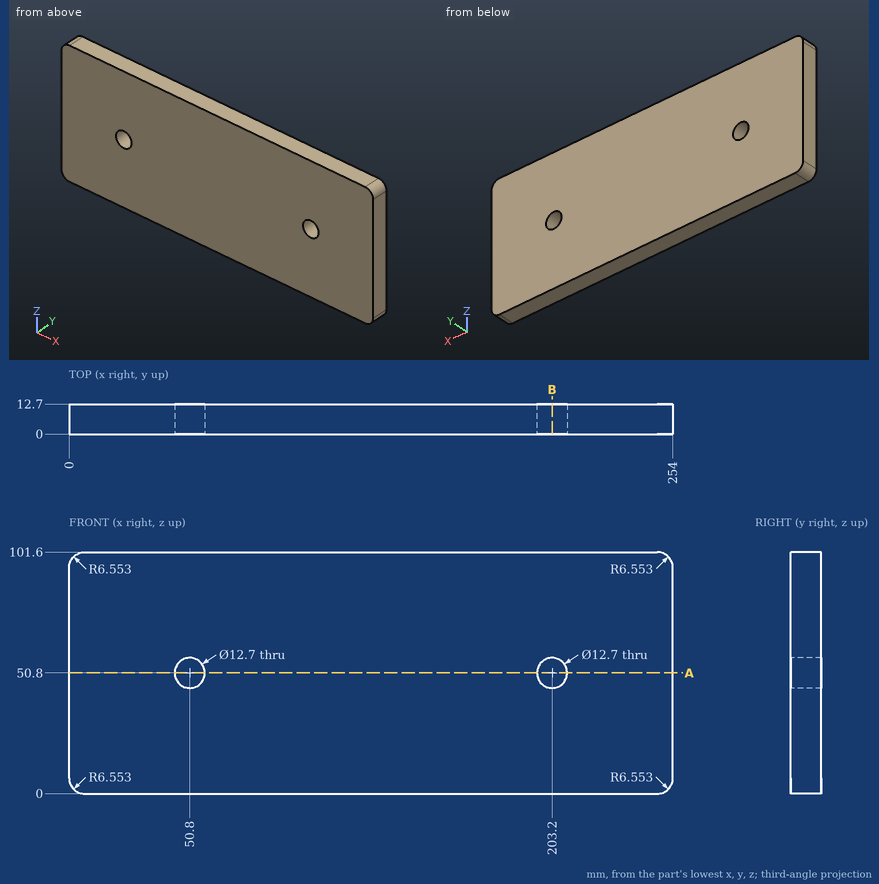
Source: three-view drawing plus pictorial views. Frame: mm from the lowest corner of the part. Round coordinates to 2 decimals unless told otherwise and drop trailing zeros. Loops run counter-clockwise (first coordinate to the right, second up) from the corner with the lowest first, then second, coordinate; pieces in that order, holes last. Notation, with made-up numbers: (2.25, -37) -> (49.25, -37) arc R18 cw to (49.25, -20) -> close; hole circle Ø11 at (-7, 55.25). An arc over 180 degrees is marked (long way). Use one line per item in the form item = value.
Item 1: Cut plane A-A on z = 50.8. Output: boundary loops of the cut face in (x, y).
Evaluation:
outline = (0, 0) -> (44.45, 0) -> (44.45, 12.7) -> (0, 12.7) -> close; (57.15, 0) -> (196.85, 0) -> (196.85, 12.7) -> (57.15, 12.7) -> close; (209.55, 0) -> (254, 0) -> (254, 12.7) -> (209.55, 12.7) -> close
Item 2: Cut plane B-B on x = 203.2. Output: boundary loops of the cut face in (y, z).
Evaluation:
outline = (0, 0) -> (12.7, 0) -> (12.7, 44.45) -> (0, 44.45) -> close; (0, 57.15) -> (12.7, 57.15) -> (12.7, 101.6) -> (0, 101.6) -> close
Item 3: Material intervals for probe 1 along X at (y, z) = (8.75, 51); probe 2 along Z at (x, y) = (203.2, 6.5); probe 3 along X at (y, z) = (1.75, 52.5), sorted ascending.
Evaluation:
probe_1 = 0 to 44.45, 57.15 to 196.85, 209.55 to 254
probe_2 = 0 to 44.45, 57.15 to 101.6
probe_3 = 0 to 44.68, 56.92 to 197.08, 209.32 to 254
Item 4: Contact query for a flat-ended pin moving along its axis: pin 1 Ø7.5 at (x, z) = (203.2, 50.8) entering from -Y. Output: stop coordinate, or through.
Evaluation:
pin_1 = through
